Work out the finished part from the listing and answer in its coordinate system (mm). Face numbers are marked on the shaded views. A direction names the side the tool comes from. Coordinates: 2 decimals unless noted, no trailing zeros. Order: outer loops, then holes, each group sorted by start corner. A loop starts at its lowest first (then second) coordinate and runs counter-clockwise, first axis right, second up. Notation, with made-up numbers: M 74.5,69 L 107.5,69 A23 cw 107.5,108 Z; hole C 69,-40 d5. An arc over 180 degrees is marked long. Use a Markdown table: item, result.
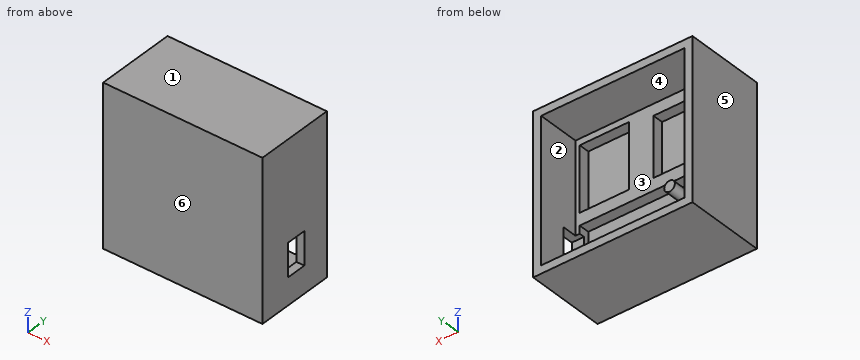
from build123d import *

# Parameters (mm, degrees)
SKETCH1_W           = 76.2
SKETCH1_H           = 76.2
BOSS_EXTRUDE1_DEPTH = 38.1
SKETCH2_W           = 51.308
SKETCH2_H           = 23.368
SKETCH2_W_2         = 23.622
SKETCH2_H_2         = 30.988
SKETCH2_W_3         = 25.7302
SKETCH2_H_3         = 28.5242
CUT_EXTRUDE3_DEPTH  = 25.4
SKETCH8_W           = 68.58
SKETCH8_H           = 68.58
SKETCH8_W_2         = 25.7302
SKETCH8_H_2         = 28.5242
SKETCH8_W_3         = 23.622
SKETCH8_H_3         = 30.988
SKETCH8_W_4         = 51.308
SKETCH8_H_4         = 23.368
CUT_EXTRUDE5_DEPTH  = 20.32
SKETCH10_W          = 15.875
SKETCH10_H          = 9.525
CUT_EXTRUDE6_DEPTH  = 20.32
CUT_EXTRUDE7_DEPTH  = 5.08
SKETCH12_R          = 2.54
BOSS_EXTRUDE2_DEPTH = 25.4


with BuildPart() as part:
    # Sketch1 → Boss-Extrude1 (new body)
    with BuildSketch(Plane(origin=(0, 0, 0), x_dir=(1, 0, 0), z_dir=(0, 1, 0))):
        Rectangle(SKETCH1_W, SKETCH1_H)
    extrude(amount=BOSS_EXTRUDE1_DEPTH)

    # Sketch2 → Cut-Extrude3 (cut)
    with BuildSketch(Plane(origin=(0, 38.1, 0), x_dir=(1, 0, 0), z_dir=(0, 1, 0))):
        with Locations((6.604, 17.272)):
            Rectangle(SKETCH2_W, SKETCH2_H)
        with Locations((20.447, -15.748)):
            Rectangle(SKETCH2_W_2, SKETCH2_H_2)
        with Locations((-15.9131, -14.5161)):
            Rectangle(SKETCH2_W_3, SKETCH2_H_3)
    extrude(amount=-CUT_EXTRUDE3_DEPTH, mode=Mode.SUBTRACT)

    # Sketch8 → Cut-Extrude5 (cut)
    with BuildSketch(Plane(origin=(0, 38.1, 0), x_dir=(1, 0, 0), z_dir=(0, 1, 0))):
        Rectangle(SKETCH8_W, SKETCH8_H)
        with Locations((-15.9131, -14.5161)):
            Rectangle(SKETCH8_W_2, SKETCH8_H_2, mode=Mode.SUBTRACT)
        with Locations((20.447, -15.748)):
            Rectangle(SKETCH8_W_3, SKETCH8_H_3, mode=Mode.SUBTRACT)
        with Locations((6.604, 17.272)):
            Rectangle(SKETCH8_W_4, SKETCH8_H_4, mode=Mode.SUBTRACT)
    extrude(amount=-CUT_EXTRUDE5_DEPTH, mode=Mode.SUBTRACT)

    # Sketch10 → Cut-Extrude6 (cut)
    with BuildSketch(Plane(origin=(38.1, 0, 0), x_dir=(0, 0, -1), z_dir=(1, 0, 0))):
        with Locations((17.272, 20.0025)):
            Rectangle(SKETCH10_W, SKETCH10_H)
    extrude(amount=-CUT_EXTRUDE6_DEPTH, mode=Mode.SUBTRACT)

    # Sketch11 → Cut-Extrude7 (cut)
    with BuildSketch(Plane(origin=(0, 17.78, 0), x_dir=(1, 0, 0), z_dir=(0, 1, 0))):
        with BuildLine():
            Line((-19.05, 28.956), (-19.05, 22.606))
            Line((-19.05, 22.606), (-22.86, 22.606))
            ThreePointArc((-22.86, 22.606), (-32.470396483, 25.781), (-22.86, 28.956))
            Line((-22.86, 28.956), (-19.05, 28.956))
        make_face()
    extrude(amount=-CUT_EXTRUDE7_DEPTH, mode=Mode.SUBTRACT)

    # Sketch12 → Boss-Extrude2 (add)
    with BuildSketch(Plane(origin=(0, 12.7, 0), x_dir=(1, 0, 0), z_dir=(0, 1, 0))):
        with Locations((-27.140733667, 25.781)):
            Circle(SKETCH12_R)
    extrude(amount=BOSS_EXTRUDE2_DEPTH)


solid = part.part
1. Section A-A on z = -12 is taken. Determine the outline of the cut face in (x, y) (3 decimals).
Answers below:
| item | result |
|---|---|
| outline | M -38.1,0 L 38.1,0 L 38.1,15.24 L 32.258,15.24 L 32.258,12.7 L -19.05,12.7 L -19.05,17.78 L -34.29,17.78 L -34.29,38.1 L -38.1,38.1 Z; M 34.29,24.765 L 38.1,24.765 L 38.1,38.1 L 34.29,38.1 Z |
2. Find the intervals of material crossed by probe 1 along X at (y, z) = (24, -26); probe 2 along Z at (x, y) = (-17.5, 13); probe 3 along X at (y, z) = (31, -12.5), in increasing order.
Answers below:
| item | result |
|---|---|
| probe 1 | -38.1 to -34.29, -29.67 to -24.61, 34.29 to 38.1 |
| probe 2 | -38.1 to -28.96, -5.59 to 0.25, 28.78 to 38.1 |
| probe 3 | -38.1 to -34.29, 34.29 to 38.1 |
3. For a pull along X with two mould halves and no side action, classify the marked faces 3, 4, 5 and 6 as +X half, -X half, draft (parallel to the pull), parting line (faces both ways), or undercut.
Answers below:
| item | result |
|---|---|
| face 3 | undercut |
| face 4 | undercut |
| face 5 | -X half |
| face 6 | draft |
4. Flat-ended cylindrical pins translate along their axes: P1, Ø7, axis at x = 19.5, z = 12.5, coming from the +Y side; P2, Ø20.5, axis at x = -11.5, z = 21.5, coming from the +Y side. Find the tip coordinate at first contact, or state that the pin passes through.
Answers below:
| item | result |
|---|---|
| P1 | y = 12.7 |
| P2 | y = 17.78 |
5. Section C-C on x = 10 is taken. Determine the outline of the cut face in (y, z).
Answers below:
| item | result |
|---|---|
| outline | M 0,-38.1 L 38.1,-38.1 L 38.1,-34.29 L 17.78,-34.29 L 17.78,-28.96 L 12.7,-28.96 L 12.7,-5.59 L 17.78,-5.59 L 17.78,0.25 L 12.7,0.25 L 12.7,31.24 L 17.78,31.24 L 17.78,34.29 L 38.1,34.29 L 38.1,38.1 L 0,38.1 Z |
6. Section B-B on y = 26.5 is taken. Determine the outline of the cut face in (x, z), then the cut area to 3 significant figures.
Answers below:
| item | result |
|---|---|
| outline | M -38.1,-38.1 L 38.1,-38.1 L 38.1,38.1 L -38.1,38.1 Z; C -27.14,-25.78 d5.08; hole M -34.29,-34.29 L 34.29,-34.29 L 34.29,34.29 L -34.29,34.29 Z |
| area | 1,120 mm² |
7. Section D-D on z = 10 is taken. Determine the outline of the cut face in (x, y).
Answers below:
| item | result |
|---|---|
| outline | M -38.1,0 L 38.1,0 L 38.1,38.1 L 34.29,38.1 L 34.29,17.78 L 32.26,17.78 L 32.26,12.7 L 8.64,12.7 L 8.64,17.78 L -3.05,17.78 L -3.05,12.7 L -28.78,12.7 L -28.78,17.78 L -34.29,17.78 L -34.29,38.1 L -38.1,38.1 Z |
8. For the marked faces 1 and 2, determine the directions among +Z, -Z, +X, -X, +Y, -Y from which every point of the face is accessible in a straight line to the end or side of a thin tool.
Answers below:
| item | result |
|---|---|
| face 1 | +Z, +X, -X, +Y, -Y |
| face 2 | +Y |
